For this review, take the finished solid that the model builds, in its own axes (mm). Face numbers are marked on the shaded views. A direction names the side the tool comes from. Coordinates: 2 decimals unless noted, no trailing zeros. Loops run counter-clockwise (first coordinate to the right, second up) from the corner with the lowest first, then second, coordinate; pieces in that order, holes last. Notation, with made-up numbers: (19.5, 77.5) - (27.5, 77.5) arc R26 ccw to (27.5, 115.5) - close; hole circle Ø9 at (-7, 54). An arc over 180 degrees is marked (long way). Use one line per item in the form item = value. Start each with the question number.
1. Machinability: for the marked faces 5, 6 and 7, which of the approach directions +Z, -Z, +X, -X, +Y, -Y give a long, thin tool a straight path to every point of the face, cutting with its end or side? Answer none if there is none.
2. Add section B-B on z = -5. Give the boundary of the cut face in (x, y).
3. Add section A-A on y = 28.5. Give the boundary of the cut face in (x, z).
4. To check wall thickness, follow probe 1 along Y at (x, z) = (-19.25, 0); probe 2 along X at (y, z) = (31, 16.5); probe 3 along Y at (x, z) = (1, 14). State the ranges of each line that lie inside material, in increasing order.
5. Add section C-C on y = 40.5. Give the boundary of the cut face in (x, z).
6. Add section D-D on x = 9. Give the boundary of the cut face in (y, z), and give its area (3 significant figures).
7. For pin 1 Ø2.5 at (y, z) = (23, -17.5) entering from +X; pin 2 Ø6.5 at (x, y) = (-21, 27) entering from +Z; pin 3 Ø10 at (x, z) = (1, 10.5) entering from -Y; pin 4 Ø4 at (x, y) = (-21.5, 28.5) entering from -Z, all flat-tipped, find the tip position at first contact; note any pin that passes through.
8. Draft analysis for pull direction Y (two halves, no side actions). For the marked faces 1, 2, 3 and 4, state which applies: +Y half, -Y half, draft (parallel to the pull), parting line (faces both ways), or undercut.
```python
from build123d import *

# Parameters (mm, degrees)
SKETCH_1_W               = 48
SKETCH_1_H               = 42
EXTRUDE_1_DEPTH          = 45
CUT_EXTRUDE_1_DEPTH      = 56.154328933
CUT_EXTRUDE_1_DEPTH_BACK = 56.154328933
SKETCH_2_W               = 34
SKETCH_2_H               = 41
CUT_EXTRUDE_2_REACH      = 71.065
SKETCH_3_R               = 10.5
CUT_EXTRUDE_3_REACH      = 67.038
SKETCH_4_R               = 13
CUT_EXTRUDE_4_REACH      = 71.065
SKETCH_5_R               = 2
CUT_EXTRUDE_5_DEPTH      = 70.065186599
CUT_EXTRUDE_6_REACH      = 71.065
HOLE_WIZARD_M3_1_D       = 2.5
HOLE_WIZARD_M3_1_DEPTH   = 16.5
HOLE_WIZARD_M3_1_TIP     = 0.751075774


with BuildPart() as part:
    # 草图1 → 凸台-拉伸1 (new body)
    with BuildSketch(Plane(origin=(0, 0, 0), x_dir=(1, 0, 0), z_dir=(0, 1, 0))):
        Rectangle(SKETCH_1_W, SKETCH_1_H)
    extrude(amount=EXTRUDE_1_DEPTH)

    # 草图2 → 切除-拉伸1 (cut, two sides: drawn at the far end of the back side and taken through both)
    with BuildSketch(Plane.XY.offset(-CUT_EXTRUDE_1_DEPTH_BACK)):
        with Locations((1, 24.5)):
            Rectangle(SKETCH_2_W, SKETCH_2_H)
    extrude(amount=CUT_EXTRUDE_1_DEPTH + CUT_EXTRUDE_1_DEPTH_BACK, mode=Mode.SUBTRACT)

    # 草图3 → 切除-拉伸2 (cut, up to next)
    with BuildSketch(Plane.ZY.offset(24), mode=Mode.PRIVATE) as cut_extrude_2_sk1:
        with Locations((0, 23)):
            Circle(SKETCH_3_R)
    cut_extrude_2_tool1 = extrude(cut_extrude_2_sk1.sketch, amount=-CUT_EXTRUDE_2_REACH, mode=Mode.PRIVATE) & part.part
    add(cut_extrude_2_tool1.solids().sort_by_distance((-24, 23, 0))[0], mode=Mode.SUBTRACT)

    # 草图4 → 切除-拉伸3 (cut, up to next)
    with BuildSketch(Plane.ZY.offset(-18), mode=Mode.PRIVATE) as cut_extrude_3_sk1:
        with Locations(Location((0, 23, 0), (0, 0, 270))):
            Circle(SKETCH_4_R)
    cut_extrude_3_tool1 = extrude(cut_extrude_3_sk1.sketch, amount=-CUT_EXTRUDE_3_REACH, mode=Mode.PRIVATE) & part.part
    add(cut_extrude_3_tool1.solids().sort_by_distance((18, 23, 0))[0], mode=Mode.SUBTRACT)

    # 草图5 → 切除-拉伸4 (cut, up to next)
    with BuildSketch(Plane(origin=(24, 0, 0), x_dir=(0, 0, -1), z_dir=(1, 0, 0)), mode=Mode.PRIVATE) as cut_extrude_4_sk1:
        with Locations((17.5, 23)):
            Circle(SKETCH_5_R)
    cut_extrude_4_tool1 = extrude(cut_extrude_4_sk1.sketch, amount=-CUT_EXTRUDE_4_REACH, mode=Mode.PRIVATE) & part.part
    # 草图5 → 切除-拉伸4 (cut, up to next)
    with BuildSketch(Plane(origin=(24, 0, 0), x_dir=(0, 0, -1), z_dir=(1, 0, 0)), mode=Mode.PRIVATE) as cut_extrude_4_sk2:
        with Locations((-17.5, 23)):
            Circle(SKETCH_5_R)
    cut_extrude_4_tool2 = extrude(cut_extrude_4_sk2.sketch, amount=-CUT_EXTRUDE_4_REACH, mode=Mode.PRIVATE) & part.part
    # 草图5 → 切除-拉伸4 (cut, up to next)
    with BuildSketch(Plane(origin=(24, 0, 0), x_dir=(0, 0, -1), z_dir=(1, 0, 0)), mode=Mode.PRIVATE) as cut_extrude_4_sk3:
        with Locations((0, 40.5)):
            Circle(SKETCH_5_R)
    cut_extrude_4_tool3 = extrude(cut_extrude_4_sk3.sketch, amount=-CUT_EXTRUDE_4_REACH, mode=Mode.PRIVATE) & part.part
    add(cut_extrude_4_tool1.solids().sort_by_distance((24, 23, -17.5))[0], mode=Mode.SUBTRACT)
    add(cut_extrude_4_tool2.solids().sort_by_distance((24, 23, 17.5))[0], mode=Mode.SUBTRACT)
    add(cut_extrude_4_tool3.solids().sort_by_distance((24, 40.5, 0))[0], mode=Mode.SUBTRACT)

    # 草图6 → 切除-拉伸5 (cut, through all)
    with BuildSketch(Plane.ZY.offset(24)):
        with BuildLine():
            ThreePointArc((0, 45), (13.033348619, 40.723764379), (21, 29.557438524))
            Line((21, 29.557438524), (21, 45))
            Line((21, 45), (0, 45))
        make_face()
        with BuildLine():
            ThreePointArc((-21, 29.557438524), (-13.033348619, 40.723764379), (0, 45))
            Line((0, 45), (-21, 45))
            Line((-21, 45), (-21, 29.557438524))
        make_face()
    extrude(amount=-CUT_EXTRUDE_5_DEPTH, mode=Mode.SUBTRACT)

    # 草图7 → 切除-拉伸6 (cut, up to next)
    with BuildSketch(Plane.ZY.offset(24), mode=Mode.PRIVATE) as cut_extrude_6_sk1:
        with BuildLine():
            Line((-17, 36.964240044), (-17, 4))
            Line((-17, 4), (-21, 4))
            Line((-21, 4), (-21, 29.557438524))
            ThreePointArc((-21, 29.557438524), (-19.357561241, 33.453938149), (-17, 36.964240044))
        make_face()
    cut_extrude_6_tool1 = extrude(cut_extrude_6_sk1.sketch, amount=-CUT_EXTRUDE_6_REACH, mode=Mode.PRIVATE) & part.part
    # 草图7 → 切除-拉伸6 (cut, up to next)
    with BuildSketch(Plane.ZY.offset(24), mode=Mode.PRIVATE) as cut_extrude_6_sk2:
        with BuildLine():
            Line((21, 29.557438524), (21, 4))
            Line((21, 4), (17, 4))
            Line((17, 4), (17, 36.964240044))
            ThreePointArc((17, 36.964240044), (19.357561241, 33.453938149), (21, 29.557438524))
        make_face()
    cut_extrude_6_tool2 = extrude(cut_extrude_6_sk2.sketch, amount=-CUT_EXTRUDE_6_REACH, mode=Mode.PRIVATE) & part.part
    add(cut_extrude_6_tool1.solids().sort_by_distance((-24, 18.988652, -18.919979))[0], mode=Mode.SUBTRACT)
    add(cut_extrude_6_tool2.solids().sort_by_distance((-24, 18.988652, 18.919979))[0], mode=Mode.SUBTRACT)

    # M3 螺纹孔1
    with Locations(Plane(origin=(21, 0, -12.5), x_dir=(0, 0, -1), z_dir=(0, -1, 0))):
        with Locations((0, 0), (-25, 0), (-25, -42), (0, -42)):
            Hole(HOLE_WIZARD_M3_1_D / 2, depth=HOLE_WIZARD_M3_1_DEPTH)
            with Locations((0, 0, -(HOLE_WIZARD_M3_1_DEPTH + HOLE_WIZARD_M3_1_TIP / 2))):  # 118° drill point
                Cone(0, HOLE_WIZARD_M3_1_D / 2, HOLE_WIZARD_M3_1_TIP, mode=Mode.SUBTRACT)


solid = part.part
```
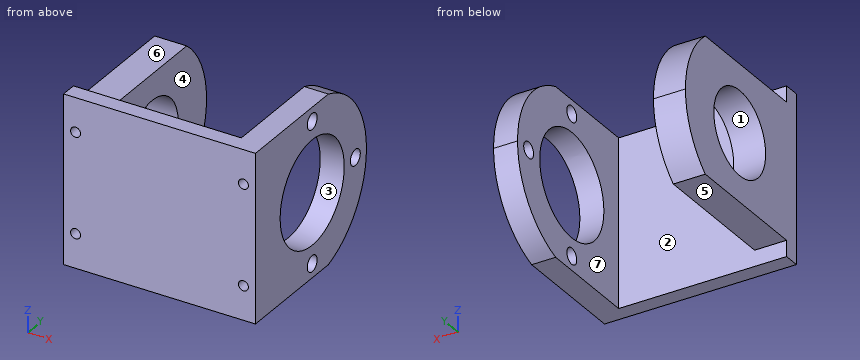
Conclusion:
q1.face_5 = -Z, -X, +Y
q1.face_6 = +Z, -X, +Y
q1.face_7 = +Z, -Z, +Y
q2.outline = (-24, 0) - (24, 0) - (24, 11) - (18, 11) - (18, 4) - (-16, 4) - (-16, 13.77) - (-24, 13.77) - close; (-24, 32.23) - (-16, 32.23) - (-16, 44.42) - (-24, 44.42) - close; (18, 35) - (24, 35) - (24, 44.42) - (18, 44.42) - close
q3.outline = (-24, -17) - (-16, -17) - (-16, -8.94) - (-24, -8.94) - close; (-24, 8.94) - (-16, 8.94) - (-16, 17) - (-24, 17) - close; (18, -21) - (24, -21) - (24, -11.78) - (18, -11.78) - close; (18, 11.78) - (24, 11.78) - (24, 21) - (18, 21) - close
q4.probe_1 = 0 to 12.5, 33.5 to 45
q4.probe_2 = -24 to -16, 18 to 24
q4.probe_3 = 0 to 4
q5.outline = (-24, -13.33) - (-16, -13.33) - (-16, 13.33) - (-24, 13.33) - close; (18, -13.33) - (24, -13.33) - (24, -2) - (18, -2) - close; (18, 2) - (24, 2) - (24, 13.33) - (18, 13.33) - close
q6.outline = (0, -21) - (4, -21) - (4, 21) - (0, 21) - close
q6.area = 168 mm^2
q7.pin_1 = -16
q7.pin_2 = 17
q7.pin_3 = 0
q7.pin_4 = -17
q8.face_1 = undercut
q8.face_2 = +Y half
q8.face_3 = undercut
q8.face_4 = draft
